from build123d import *

# Parameters (mm, degrees)
SKETCH1_R           = 23.8125
BOSS_EXTRUDE1_DEPTH = 10.16
SKETCH2_R           = 16.1925
SKETCH2_R_2         = 10.16
CUT_EXTRUDE1_DEPTH  = 3.175
SKETCH3_R           = 16.1925
SKETCH3_R_2         = 10.16
CUT_EXTRUDE2_DEPTH  = 3.175
SKETCH4_R           = 10.16
CUT_EXTRUDE3_DEPTH  = 1.27
SKETCH7_R           = 10.16
CUT_EXTRUDE5_DEPTH  = 1.27
FILLET1_R           = 1.27


with BuildPart() as part:
    # Sketch1 → Boss-Extrude1 (new body)
    with BuildSketch(Plane.XY):
        Circle(SKETCH1_R)
        Polygon((3.569234353, -6.4049902), (7.331501401, -0.111447478), (3.762267048, 6.293542722), (-3.569234353, 6.4049902), (-7.331501401, 0.111447478), (-3.762267048, -6.293542722), align=None, mode=Mode.SUBTRACT)
    extrude(amount=BOSS_EXTRUDE1_DEPTH)

    # Sketch2 → Cut-Extrude1 (cut)
    with BuildSketch(Plane.XY.offset(10.16)):
        Circle(SKETCH2_R)
        Circle(SKETCH2_R_2, mode=Mode.SUBTRACT)
    extrude(amount=-CUT_EXTRUDE1_DEPTH, mode=Mode.SUBTRACT)

    # Sketch3 → Cut-Extrude2 (cut)
    with BuildSketch(Plane(origin=(0, 0, 0), x_dir=(-1, 0, 0), z_dir=(0, 0, -1))):
        Circle(SKETCH3_R)
        Circle(SKETCH3_R_2, mode=Mode.SUBTRACT)
    extrude(amount=-CUT_EXTRUDE2_DEPTH, mode=Mode.SUBTRACT)

    # Sketch4 → Cut-Extrude3 (cut)
    with BuildSketch(Plane(origin=(0, 0, 0), x_dir=(-1, 0, 0), z_dir=(0, 0, -1))):
        Circle(SKETCH4_R)
    extrude(amount=-CUT_EXTRUDE3_DEPTH, mode=Mode.SUBTRACT)

    # Sketch7 → Cut-Extrude5 (cut)
    with BuildSketch(Plane.XY.offset(10.16)):
        Circle(SKETCH7_R)
    extrude(amount=-CUT_EXTRUDE5_DEPTH, mode=Mode.SUBTRACT)

    # Fillet1
    fillet1_edges = [part.edges().sort_by_distance(p)[0] for p in [
        (-16.1925, 0, 6.985),
        (-10.16, 0, 6.985),
        (16.1925, 0, 3.175),
        (10.16, 0, 3.175),
    ]]
    fillet(fillet1_edges, radius=FILLET1_R)


solid = part.part
Input: part model. Units: mm. Frame: model coordinates. A direction names the side the tool comes from. Coordinates: 2 decimals unless noted, no trailing zeros. Loops run counter-clockwise (first coordinate to the right, second up) from the corner with the lowest first, then second, coordinate; pieces in that order, holes last. Notation, with made-up numbers: (34, 50) - (92, 50) arc R24 ccw to (92, 70) - close; hole circle Ø9 at (-13, 59). An arc over 180 degrees is marked (long way). Answer in a Markdown table with one row per item. Add a question column.
Item 1: Section query D-D on y = 20.5. Return the cut outline in (x, z), then the cut area to 3 significant figures.
Item 2: Line query: line 1 along Y through (x, z) = (0, 0.9); line 2 along X through (y, z) = (-1, 2); line 3 along Y through (x, z) = (6, 2.5). Output: solid intervals per line, ascending. Write a range as [from, to].
Item 3: Contact query for flat-ended pins moving along their axis: P1, Ø1.5, axis at x = 11.5, z = 6.5, coming from the -Y side; P2, Ø1, axis at x = -6, z = 8, coming from the -Y side; P3, Ø5, axis at y = 14, z = 7, coming from the +X side. Output: stop coordinate, or through.
Item 4: Section query C-C on x = -21. Return the cut outline in (y, z).
Item 5: Section query A-A on z = 5. Return the cut outline in (x, y) (1 decimal), then the cut area to 3 significant figures.
Item 6: Access query for faces 4 (the flat face through (5, -16, 0)), 5 (the flat face through (8, -9, 6.985)), 6 (the flat face through (-5.424, 3.302, 5.027)), 7 (the flat face through (0, -7, 1.27)). Directions: +Z, -Z, +X, -X, +Y, -Y. A direction counts if a zero-diameter tool reaches every point of the face in a straight line with its end or side. Return the directions, or none.
Item 7: Mould query, pull axis Y, two halves, no side actions, for faces 1 (the cylindrical face through (-18.897, -14.49, 5.009)), 2 (the flat face through (0, -7, 8.89)), 3 (the flat face through (5, -16, 10.16)). Classes: released by +Y, released by -Y, zero draft, split by the parting line, or undercut.
Recorded:
| question | item | result |
|---|---|---|
| 1 | outline | (-12.12, 0) - (12.12, 0) - (12.12, 10.16) - (-12.12, 10.16) - close |
| 1 | area | 246 mm^2 |
| 2 | line 1 | [-23.81, -16.19], [16.19, 23.81] |
| 2 | line 2 | [-23.79, -16.16], [-10.11, -6.71], [6.8, 10.11], [16.16, 23.79] |
| 2 | line 3 | [-23.04, -14.88], [-8.38, -2.34], [2.28, 8.38], [14.88, 23.04] |
| 3 | P1 | y = -21.25 |
| 3 | P2 | y = -23.17 |
| 3 | P3 | x = 20.85 |
| 4 | outline | (-11.23, 0) - (11.23, 0) - (11.23, 10.16) - (-11.23, 10.16) - close |
| 5 | outline | circle Ø47.6 at (0, 0); hole (-7.3, 0.1) - (-3.8, -6.3) - (3.6, -6.4) - (7.3, -0.1) - (3.8, 6.3) - (-3.6, 6.4) - close |
| 5 | area | 1,640 mm^2 |
| 6 | face 4 | -Z, +X, -X, +Y, -Y |
| 6 | face 5 | +Z |
| 6 | face 6 | +Z, -Z |
| 6 | face 7 | -Z |
| 7 | face 1 | split by the parting line |
| 7 | face 2 | undercut |
| 7 | face 3 | zero draft |
